The listing builds one solid part. Answer for the finished solid, in the listing's coordinates (mm). Face numbers are marked on the shaded views. A direction names the side the tool comes from. Coordinates: 2 decimals unless noted, no trailing zeros. Loops run counter-clockwise (first coordinate to the right, second up) from the corner with the lowest first, then second, coordinate; pieces in that order, holes last. Notation, with made-up numbers: (-17.75, 37) - (27.25, 37) arc R17 ccw to (27.25, 49) - close; hole circle Ø8 at (7, 61). An arc over 180 degrees is marked (long way). Use one line per item in the form item = value. Start each with the question number.
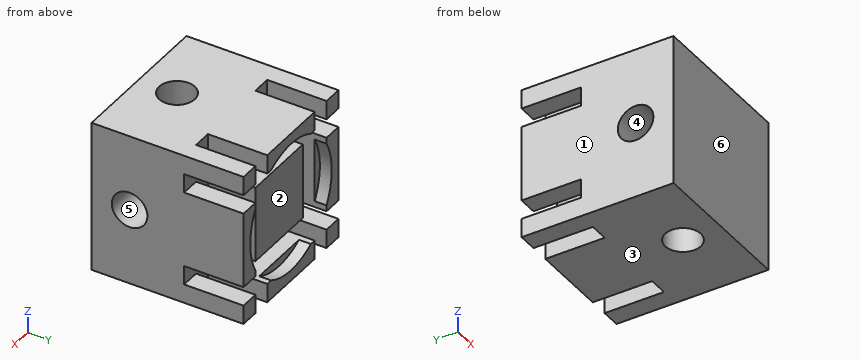
```python
from build123d import *

# Parameters (mm, degrees)
SKETCH2_W           = 16.256
SKETCH2_H           = 16.256
BOSS_EXTRUDE1_DEPTH = 16.256
SKETCH3_R           = 6.985
CUT_EXTRUDE1_DEPTH  = 1.27
SKETCH4_W           = 2.032
SKETCH4_H           = 16.256
SKETCH4_W_2         = 16.256
SKETCH4_H_2         = 2.032
CUT_EXTRUDE3_DEPTH  = 6.35
SKETCH7_R           = 1.905
CUT_EXTRUDE5_DEPTH  = 23.172323288
SKETCH8_R           = 1.905
CUT_EXTRUDE6_DEPTH  = 27.26414042


with BuildPart() as part:
    # Sketch2 → Boss-Extrude1 (new body)
    with BuildSketch(Plane.XY):
        with Locations((0, 4.572)):
            Rectangle(SKETCH2_W, SKETCH2_H)
    extrude(amount=-BOSS_EXTRUDE1_DEPTH)

    # Sketch3 → Cut-Extrude1 (cut)
    with BuildSketch(Plane(origin=(0, 12.7, 0), x_dir=(1, 0, 0), z_dir=(0, 1, 0))):
        with Locations(Location((0, 8.128, 0), (0, 0, 270))):
            Circle(SKETCH3_R)
    extrude(amount=-CUT_EXTRUDE1_DEPTH, mode=Mode.SUBTRACT)

    # Sketch4 → Cut-Extrude3 (cut)
    with BuildSketch(Plane(origin=(0, 12.7, 0), x_dir=(1, 0, 0), z_dir=(0, 1, 0))):
        with Locations((-5.08, 8.128)):
            Rectangle(SKETCH4_W, SKETCH4_H)
        with Locations((5.08, 8.128)):
            Rectangle(SKETCH4_W, SKETCH4_H)
        with Locations((0, 13.208)):
            Rectangle(SKETCH4_W_2, SKETCH4_H_2)
        with Locations((0, 3.048)):
            Rectangle(SKETCH4_W_2, SKETCH4_H_2)
    extrude(amount=-CUT_EXTRUDE3_DEPTH, mode=Mode.SUBTRACT)

    # Sketch7 → Cut-Extrude5 (cut, through all)
    with BuildSketch(Plane.XY):
        with Locations((0, 0.508)):
            Circle(SKETCH7_R)
    extrude(amount=-CUT_EXTRUDE5_DEPTH, mode=Mode.SUBTRACT)

    # Sketch8 → Cut-Extrude6 (cut, through all)
    with BuildSketch(Plane(origin=(8.128, 0, 0), x_dir=(0, 0, -1), z_dir=(1, 0, 0))):
        with Locations(Location((8.128, 0.508, 0), (0, 0, 90))):
            Circle(SKETCH8_R)
    extrude(amount=-CUT_EXTRUDE6_DEPTH, mode=Mode.SUBTRACT)


solid = part.part
```
(1) A cutting plane is placed at C-C (z = -5). Determine the outline of the cut face in (x, y) (3 decimals).
(2) Find the intervals of material crossed by probe 1 along Z at (x, y) = (-1.25, 7); probe 2 along X at (y, z) = (10.5, -8); probe 3 along Y at (x, z) = (0, -11.75), in increasing order. Write a range as from..to.
(3) Determine the mould class of the marked faces 3, 4, 5 and 6 for opening direction Y: +Y half, -Y half, draft (parallel to the pull), parting line (faces both ways), or undercut.
(4) A cutting plane is placed at B-B (y = -0.75). Determine the outline of the cut face in (x, z).
(5) For the marked faces 1 and 2, determine the directions among +Z, -Z, +X, -X, +Y, -Y from which every point of the face is accessible in a straight line to the end or side of a thin tool.
(6) This flat-tipped pin is pushed along its axis until it touches: pin 1 Ø2 at (x, z) = (3.5, -8) entering from +Y. Where does it stop, or does it pass through?
(7) A cutting plane is placed at D-D (x = 0.5). Determine the outline of the cut face in (y, z) (3 decimals), then the cut area to 3 significant figures.
(8) A cutting plane is placed at A-A (x = -4.5). Determine the outline of the cut face in (y, z) (3 decimals).
Evaluation:
q1.outline = (-8.128, -3.556) - (8.128, -3.556) - (8.128, 12.7) - (6.245, 12.7) - (6.245, 11.43) - (6.096, 11.43) - (6.096, 6.35) - (4.064, 6.35) - (4.064, 11.43) - (-4.064, 11.43) - (-4.064, 6.35) - (-6.096, 6.35) - (-6.096, 11.43) - (-6.245, 11.43) - (-6.245, 12.7) - (-8.128, 12.7) - close; hole circle Ø3.81 at (0, 0.508)
q2.probe_1 = -16.26..-14.22, -12.19..-4.06, -2.03..0
q2.probe_2 = -8.13..-6.1, -4.06..4.06, 6.1..8.13
q2.probe_3 = -3.56..-1.4, 2.41..11.43
q3.face_3 = draft
q3.face_4 = undercut
q3.face_5 = undercut
q3.face_6 = -Y half
q4.outline = (-8.13, -16.26) - (-1.43, -16.26) - (-1.43, -9.56) - (-8.13, -9.56) - close; (-8.13, -6.7) - (-1.43, -6.7) - (-1.43, 0) - (-8.13, 0) - close; (1.43, -16.26) - (8.13, -16.26) - (8.13, -9.56) - (1.43, -9.56) - close; (1.43, -6.7) - (8.13, -6.7) - (8.13, 0) - (1.43, 0) - close
q5.face_1 = +Z, -Z, -X, +Y, -Y
q5.face_2 = +Y
q6.pin_1 = 11.43
q7.outline = (-3.556, -16.256) - (-1.33, -16.256) - (-1.33, -8.628) arc R1.905 cw to (-1.33, -7.628) - (-1.33, 0) - (-3.556, 0) - close; (2.346, -16.256) - (12.7, -16.256) - (12.7, -15.095) - (11.43, -15.095) - (11.43, -14.224) - (6.35, -14.224) - (6.35, -12.192) - (11.43, -12.192) - (11.43, -4.064) - (6.35, -4.064) - (6.35, -2.032) - (11.43, -2.032) - (11.43, -1.161) - (12.7, -1.161) - (12.7, 0) - (2.346, 0) - (2.346, -7.628) arc R1.905 cw to (2.346, -8.628) - close
q7.area = 166 mm^2
q8.outline = (-3.556, -16.256) - (6.35, -16.256) - (6.35, 0) - (-3.556, 0) - close; hole circle Ø3.81 at (0.508, -8.128)
